Read the model definition and answer for the solid it produces. Units are mm, in the model's axes. Face numbers are marked on the shaded views. A direction names the side the tool comes from. Coordinates: 2 decimals unless noted, no trailing zeros. Write each loop counter-clockwise with the first axis right and the second up, starting at its lowest first coordinate (ties: lowest second). Pieces come first, ordered by that corner, then holes. Notation, with made-up numbers: (80, -4.5) - (100, -4.5) arc R13 cw to (100, 14.5) - close; hole circle Ø5 at (37, 46.25). An arc over 180 degrees is marked (long way). Use a Markdown table: item, result.
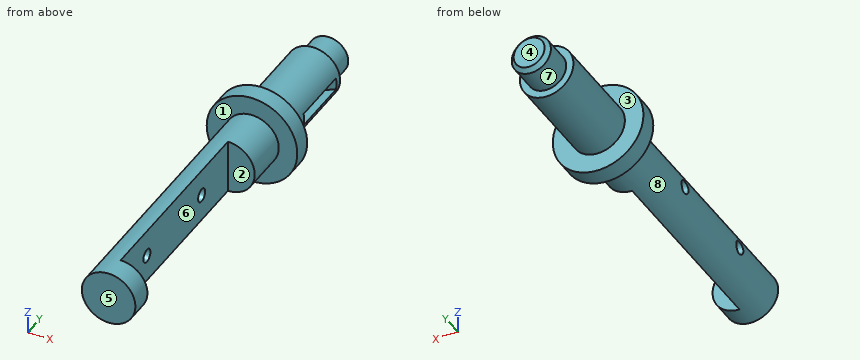
from build123d import *

# Parameters (mm, degrees)
CHAMFER1_SIZE           = 1
CUT_EXTRUDE2_DEPTH      = 103.685198544
CUT_EXTRUDE2_DEPTH_BACK = 103.685198544
SKETCH2_W               = 13.680212399
SKETCH2_H               = 49
SKETCH3_R               = 8
CUT_EXTRUDE3_DEPTH      = 1.5
CUT_EXTRUDE4_DEPTH      = 103.685198544
CUT_EXTRUDE4_DEPTH_BACK = 103.685198544
SKETCH7_R               = 1.6


with BuildPart() as part:
    # Sketch1 → Revolve1 (revolve)
    with BuildSketch(Plane.XY, mode=Mode.PRIVATE) as revolve1_sk:
        Polygon((0, 0), (6.5, 0), (6.5, 65.5), (11, 65.5), (11, 70), (6.5, 70), (6.5, 93.5), (4.75, 93.5), (4.75, 101.5), (0, 101.5), align=None)
    revolve(revolve1_sk.sketch.rotate(Axis((0, 101.5, 0), (0, -1, 0)), 180), axis=Axis((0, 101.5, 0), (0, -1, 0)))

    # Chamfer1
    chamfer1_edges = [part.edges().sort_by_distance(p)[0] for p in [
        (4.75, 101.5, 0),
    ]]
    chamfer(chamfer1_edges, length=CHAMFER1_SIZE)

    # Sketch2 → Cut-Extrude2 (cut, two sides: drawn at the far end of the back side and taken through both)
    with BuildSketch(Plane.XY.offset(-CUT_EXTRUDE2_DEPTH_BACK)):
        with Locations((6.8401062, 30)):
            Rectangle(SKETCH2_W, SKETCH2_H)
    extrude(amount=CUT_EXTRUDE2_DEPTH + CUT_EXTRUDE2_DEPTH_BACK, mode=Mode.SUBTRACT)

    # Sketch3 → Cut-Extrude3 (cut, symmetric)
    with BuildSketch(Plane.XY):
        with Locations((9.5, 84.5)):
            Circle(SKETCH3_R)
    extrude(amount=CUT_EXTRUDE3_DEPTH, both=True, mode=Mode.SUBTRACT)

    # Sketch7 → Cut-Extrude4 (cut, two sides: drawn at the far end of the back side and taken through both)
    with BuildSketch(Plane(origin=(0, 0, 0), x_dir=(0, 0, -1), z_dir=(1, 0, 0)).offset(-CUT_EXTRUDE4_DEPTH_BACK)):
        with Locations(Location((0, 42.5, 0), (0, 0, 270))):
            Circle(SKETCH7_R)
        with Locations(Location((0, 17.5, 0), (0, 0, 270))):
            Circle(SKETCH7_R)
    extrude(amount=CUT_EXTRUDE4_DEPTH + CUT_EXTRUDE4_DEPTH_BACK, mode=Mode.SUBTRACT)


solid = part.part
(1) For the marked faces 4, 5, 6, 7 and 8, determine the directions among +Z, -Z, +X, -X, +Y, -Y from which every point of the face is accessible in a straight line to the end or side of a thin tool.
Report:
| item | result |
|---|---|
| face 4 | +Z, -Z, +X, -X, +Y |
| face 5 | +Z, -Z, +X, -X, -Y |
| face 6 | +Z, -Z, +X |
| face 7 | +Y |
| face 8 | -Y |
(2) A cutting plane is placed at C-C, the plane y = 14.5. Write down the section's boundary in (x, z).
Report:
| item | result |
|---|---|
| outline | (0, -6.5) - (0, 6.5) arc R6.5 ccw to start |
(3) A cutting plane is placed at B-B, the plane y = 42.5. Write down the section's boundary in (x, z), and give its area (3 significant figures).
Report:
| item | result |
|---|---|
| outline | (-6.3, -1.6) arc R6.5 ccw to (0, -6.5) - (0, -1.6) - close; (-6.3, 1.6) - (0, 1.6) - (0, 6.5) arc R6.5 ccw to start |
| area | 45.8 mm² |
(4) A cutting plane is placed at A-A, the plane z = 0. Count the separate pieces of the cut face and the enclosed holes in it, and give its area (3 significant figures).
Report:
| item | result |
|---|---|
| separate pieces | 3 |
| enclosed holes | 0 |
| area | 917 mm² |
(5) Straight lines are drawn through the part: L1, parallel to Y at x = 1.75, z = 2.5; L2, parallel to Y at x = 3.5, z = -3.5; L3, parallel to Y at x = -7.25, z = 2. For each, find the intervals that lie inside material, in ascending order.
Report:
| item | result |
|---|---|
| L1 | y = 0 to 5.5, 54.5 to 101.5 |
| L2 | y = 0 to 5.5, 54.5 to 93.5 |
| L3 | y = 65.5 to 70 |
(6) The mould has two halves that part along Y. Classify the marked faces 1, 2 and 3: pulls with the +Y half, pulls with the -Y half, needs draft (parallel to the pull), parting line crosses it, or undercut.
Report:
| item | result |
|---|---|
| face 1 | pulls with the -Y half |
| face 2 | undercut |
| face 3 | pulls with the +Y half |
(7) Each of these flat-tipped pins is pushed along its axis until it touches: P1, Ø2.5, axis at x = 4, y = 86.5, coming from the +Z side; P2, Ø1.5, axis at x = 5, z = 3.5, coming from the +Y side; P3, Ø3, axis at y = 46, z = 7.5, coming from the +X side. Where does it stop, or does it pass through?
Report:
| item | result |
|---|---|
| P1 | stops at z = 5.89 |
| P2 | stops at y = 93.5 |
| P3 | stops at x = 0 |
